```python
from build123d import *

# Parameters (mm, degrees)
SKETCH1_W           = 69
SKETCH1_H           = 11
BOSS_EXTRUDE1_DEPTH = 127
FILLET1_R           = 5.5
SKETCH2_R           = 0.730138729
SKETCH2_W           = 13.16276312
SKETCH2_H           = 5.0626012
SKETCH2_W_2         = 8.505170017
SKETCH2_H_2         = 2.02504048
CUT_EXTRUDE1_DEPTH  = 5
SKETCH3_R           = 0.530138729
BOSS_EXTRUDE2_DEPTH = 5


with BuildPart() as part:
    # Sketch1 → Boss-Extrude1 (new body)
    with BuildSketch(Plane(origin=(0, 0, 0), x_dir=(1, 0, 0), z_dir=(0, 1, 0))):
        with Locations((34.5, 5.5)):
            Rectangle(SKETCH1_W, SKETCH1_H)
    extrude(amount=BOSS_EXTRUDE1_DEPTH)

    # Fillet1
    fillet1_edges = [part.edges().sort_by_distance(p)[0] for p in [
        (69, 63.5, 0),
        (69, 63.5, -11),
        (0, 63.5, -11),
        (0, 63.5, 0),
    ]]
    fillet(fillet1_edges, radius=FILLET1_R - 0.0001)  # a hair under: the kernel refuses the full size

    # Sketch2 → Cut-Extrude1 (cut)
    with BuildSketch(Plane(origin=(0, 127, 0), x_dir=(1, 0, 0), z_dir=(0, 1, 0))):
        with Locations(Location((36.27191042, 5.5, 0), (0, 0, 270))):
            Circle(SKETCH2_R)
        with Locations(Location((39.27191042, 5.5, 0), (0, 0, 270))):
            Circle(SKETCH2_R)
        with Locations(Location((42.27191042, 5.5, 0), (0, 0, 270))):
            Circle(SKETCH2_R)
        with Locations(Location((45.27191042, 5.5, 0), (0, 0, 270))):
            Circle(SKETCH2_R)
        with Locations((10.756400371, 5.5)):
            Rectangle(SKETCH2_W, SKETCH2_H)
        with Locations((26.045455995, 5.5)):
            Rectangle(SKETCH2_W_2, SKETCH2_H_2)
        with BuildLine():
            Line((55.003534861, 7.069406372), (63.913712973, 7.069406372))
            ThreePointArc((63.913712973, 7.069406372), (65.483119345, 5.5), (63.913712973, 3.930593628))
            Line((63.913712973, 3.930593628), (55.003534861, 3.930593628))
            ThreePointArc((55.003534861, 3.930593628), (53.434128489, 5.5), (55.003534861, 7.069406372))
        make_face()
    extrude(amount=-CUT_EXTRUDE1_DEPTH, mode=Mode.SUBTRACT)

    # Sketch3 → Boss-Extrude2 (add)
    with BuildSketch(Plane(origin=(0, 122, 0), x_dir=(1, 0, 0), z_dir=(0, 1, 0))):
        with Locations(Location((36.27191042, 5.5, 0), (0, 0, 90))):
            Circle(SKETCH3_R)
        with Locations(Location((39.27191042, 5.5, 0), (0, 0, 90))):
            Circle(SKETCH3_R)
        with Locations(Location((42.27191042, 5.5, 0), (0, 0, 90))):
            Circle(SKETCH3_R)
        with Locations(Location((45.27191042, 5.5, 0), (0, 0, 90))):
            Circle(SKETCH3_R)
        with BuildLine():
            Line((55.003534861, 4.130593628), (63.913712973, 4.130593628))
            ThreePointArc((63.913712973, 4.130593628), (65.283119345, 5.5), (63.913712973, 6.869406372))
            Line((63.913712973, 6.869406372), (55.003534861, 6.869406372))
            ThreePointArc((55.003534861, 6.869406372), (53.634128489, 5.5), (55.003534861, 4.130593628))
        make_face()
    extrude(amount=BOSS_EXTRUDE2_DEPTH)


solid = part.part
```
The model under review builds one solid part; all positions refer to its coordinate system, in mm. A direction names the side the tool comes from. Coordinates: 2 decimals unless noted, no trailing zeros. Order: outer loops, then holes, each group sorted by start corner. A loop starts at its lowest first (then second) coordinate and runs counter-clockwise, first axis right, second up. Notation, with made-up numbers: (41.25, 46) -> (96.25, 46) arc R28 ccw to (96.25, 78) -> close; hole circle Ø10 at (-4.5, 26). An arc over 180 degrees is marked (long way). Answer in a Markdown table with one row per item. Add a question column.
Item 1: Machinability: for faces 5 (the flat face through (11, 122, -6)), 6 (the cylindrical face through (1.57, 64.39, -1.65)), which of the approach directions +Z, -Z, +X, -X, +Y, -Y give a long, thin tool a straight path to every point of the face, cutting with its end or side? Answer none if there is none.
Item 2: To check wall thickness, follow probe 1 along X at (y, z) = (119, -6); probe 2 along Y at (x, z) = (12, -8); probe 3 along X at (y, z) = (17, -9). State the ranges of each line that lie inside material, in increasing order.
Item 3: Clearance check with flat-ended pins moving along their axes: pin 1 (1 mm diameter, centred on y = 26, z = -9.5, fed in from +X); pin 2 (2 mm diameter, centred on x = 11.5, z = -5, fed in from +Y). State where each tip first meets the part, or that it passes through.
Item 4: We need section B-B on x = 12.5. Write out the cut boundary in (y, z).
Item 5: Mouldability with a two-part tool opening along Z and no side actions: class faces 1 (the cylindrical face through (65.483, 124.535, -5.535)), 2 (the flat face through (59, 124, -4.131)), 3 (the flat face through (34, 63, -11)), 4 (the flat face through (34, 63, 0)) as +Z half, -Z half, draft (parallel to the pull), parting line (faces both ways), or undercut.
Final values:
| question | item | result |
|---|---|---|
| 1 | face 5 | +Y |
| 1 | face 6 | +Z, -X, +Y, -Y |
| 2 | probe 1 | x = 0.02 to 68.98 |
| 2 | probe 2 | y = 0 to 122 |
| 2 | probe 3 | x = 1.26 to 67.74 |
| 3 | pin 1 | stops at x = 67.74 |
| 3 | pin 2 | stops at y = 122 |
| 4 | outline | (0, -11) -> (127, -11) -> (127, -8.03) -> (122, -8.03) -> (122, -2.97) -> (127, -2.97) -> (127, 0) -> (0, 0) -> close |
| 5 | face 1 | undercut |
| 5 | face 2 | undercut |
| 5 | face 3 | -Z half |
| 5 | face 4 | +Z half |
